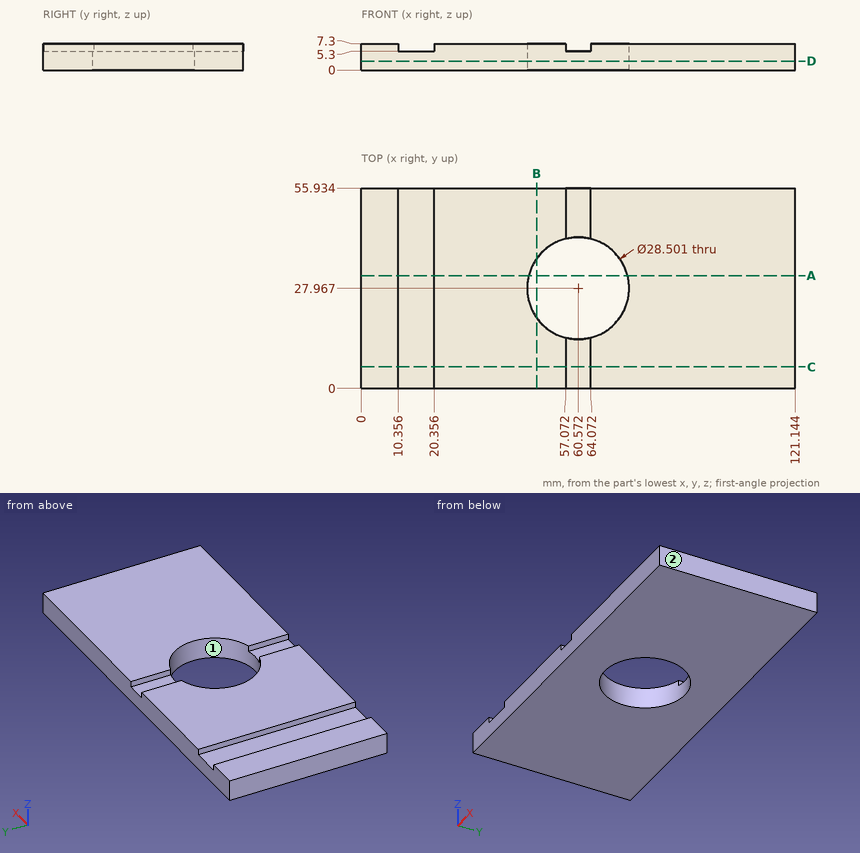
Here's the drawing with two shaded views (mm, measured from the low corner). I have some questions. Round coordinates to 2 decimals unless told otherwise and drop trailing zeros. Write each loop counter-clockwise with the first axis right and the second up, starting at its lowest first coordinate (ties: lowest second). Pieces come first, ordered by that corner, then holes.
(1) Suppose I cut it at B-B on x = 49. Write out the boundary of the cut face in (y, z), and give its area (3 significant figures).
Findings below:
outline: (0, 0) - (19.65, 0) - (19.65, 7.3) - (0, 7.3) - close; (36.28, 0) - (55.93, 0) - (55.93, 7.3) - (36.28, 7.3) - close
area: 287 mm2
(2) Suppose I cut it at C-C on y = 6. Write out the boundary of the cut face in (x, z).
Findings below:
outline: (0, 0) - (121.14, 0) - (121.14, 7.3) - (64.07, 7.3) - (64.07, 5.3) - (57.07, 5.3) - (57.07, 7.3) - (20.36, 7.3) - (20.36, 5.3) - (10.36, 5.3) - (10.36, 7.3) - (0, 7.3) - close
(3) Suppose I cut it at A-A on y = 31.5. Write out the boundary of the cut face in (x, z), and give its area (3 significant figures).
Findings below:
outline: (0, 0) - (46.77, 0) - (46.77, 7.3) - (20.36, 7.3) - (20.36, 5.3) - (10.36, 5.3) - (10.36, 7.3) - (0, 7.3) - close; (74.38, 0) - (121.14, 0) - (121.14, 7.3) - (74.38, 7.3) - close
area: 663 mm2
(4) For pin 1 (8 mm diameter, centred on x = 14.5, y = 20, fed in from +Z), with a flat end and sliding along its axis, tell me the tip position at first contact or that it passes through.
Findings below:
pin 1: stops at z = 5.3
(5) If I drill on probe 1 along X at (y, z) = (12, 5.75); probe 2 along X at (y, z) = (26.5, 6); probe 3 along Z at (x, y) = (10.5, 52.5), over which ranges is the centre line in solid material (lowest first)?
Findings below:
probe 1: x = 0 to 10.36, 20.36 to 57.07, 64.07 to 121.14
probe 2: x = 0 to 10.36, 20.36 to 46.4, 74.75 to 121.14
probe 3: z = 0 to 5.3
(6) Suppose I cut it at D-D on z = 2.5. Write out the boundary of the cut face in (x, y).
Findings below:
outline: (0, 0) - (121.14, 0) - (121.14, 55.93) - (0, 55.93) - close; hole circle Ø28.5 at (60.57, 27.97)
(7) Thinking about a two-plate mould opening in Y: for the marked faces 1 and 2, which applies, +Y half, -Y half, draft (parallel to the pull), parting line (faces both ways), or undercut?
Findings below:
face 1: undercut
face 2: draft
